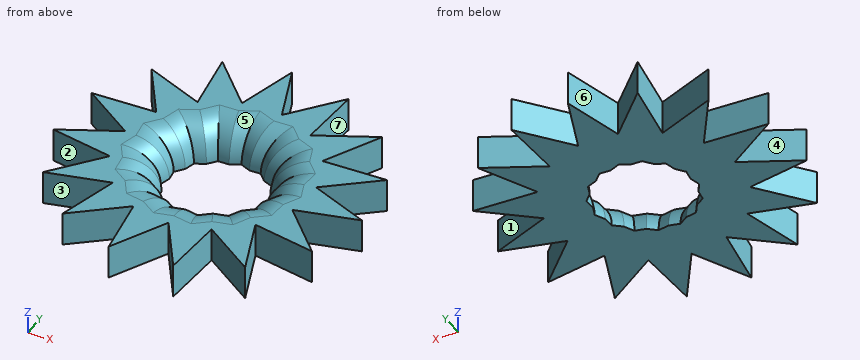
from build123d import *

# Parameters (mm, degrees)
F1_DEPTH = 5.08
F2_R     = 5.07999


# Not quite as in the source:
# - a fillet or chamfer is up to 0.001 mm smaller than in the source, because OpenCascade refuses the exact size


with BuildPart() as f1:
    # F0 (on Top) → F1 (new body)
    with BuildSketch(Plane.XY):
        Polygon((-21.999723834, 5.8521262697), (-14.0514369357, 0.7108895722), (-10.1598827967, 2.7026210629), (-12.5474815477, 6.3646642291), align=None)
        Polygon((-22.4780219717, -3.6019104497), (-13.1257712241, -5.0658043501), (-10.3807697977, -1.6634294271), (-14.0514369357, 0.7108895722), align=None)
        Polygon((-19.0696659041, -12.4331441299), (-9.930540424, -9.9665746788), (-8.8067273944, -5.7418578572), (-13.1257712241, -5.0658043501), align=None)
        Polygon((-9.930540424, -9.9665746788), (-12.3639913592, -19.1145742385), (-5.0182289685, -13.144033702), (-5.7099218179, -8.8274669008), align=None)
        Polygon((-1.6258188862, -10.3867267222), (-5.0182289685, -13.144033702), (-3.5204703849, -22.4909208108), (0.7617798649, -14.0487698884), align=None)
        Polygon((2.7394029011, -10.1500271328), (0.7617798649, -14.0487698884), (5.9317719013, -21.9783828513), (6.4100700391, -12.524346132), align=None)
        Polygon((6.6309570401, -8.1582956421), (6.4100700391, -12.524346132), (14.3583569374, -17.6655828295), (10.9500008698, -8.8343491493), align=None)
        Polygon((9.3759584665, -4.7559207191), (10.9500008698, -8.8343491493), (20.3022516175, -10.2982430497), (13.5965770725, -3.6168129411), align=None)
        Polygon((10.4997714961, -0.5312038976), (13.5965770725, -3.6168129411), (22.7357025527, -1.15024349), (13.8921815784, 2.2261030823), align=None)
        Polygon((9.8080786466, 3.7853629037), (13.8921815784, 2.2261030823), (21.2379439691, 8.1966436188), (11.7857016829, 7.6841056593), align=None)
        Polygon((7.6413668966, 11.8134565599), (7.4204798956, 7.44740607), (11.7857016829, 7.6841056593), (16.0679519327, 16.1262565817), align=None)
        Polygon((8.1196650343, 21.2674932792), (2.1757703543, 13.9001534994), (3.7498127576, 9.8217250692), (7.6413668966, 11.8134565599), align=None)
        Polygon((-1.2325857133, 22.7313871796), (-3.6660366485, 13.5833876199), (-0.5692310721, 10.4977785763), (2.1757703543, 13.9001534994), align=None)
        Polygon((-8.8739526099, 10.9179306197), (-4.7898496782, 9.3586707984), (-3.6660366485, 13.5833876199), (-10.3717111935, 20.2648177285), align=None)
        Polygon((-17.7174735842, 14.294277192), (-12.5474815477, 6.3646642291), (-8.1822597605, 6.6013638185), (-8.8739526099, 10.9179306197), align=None)
        Polygon((-12.5474815477, 6.3646642291), (-10.1598827967, 2.7026210629), (-7.7547700697, 3.9335788206), (-8.1822597605, 6.6013638185), align=None)
        Polygon((-14.0514369357, 0.7108895722), (-10.3807697977, -1.6634294271), (-8.684265617, 0.4393539178), (-10.1598827967, 2.7026210629), align=None)
        Polygon((-13.1257712241, -5.0658043501), (-8.8067273944, -5.7418578572), (-8.112172745, -3.1308392687), (-10.3807697977, -1.6634294271), align=None)
        Polygon((-8.8067273944, -5.7418578572), (-9.930540424, -9.9665746788), (-5.7099218179, -8.8274669008), (-6.1374115087, -6.1596819029), align=None)
        Polygon((-5.7099218179, -8.8274669008), (-5.0182289685, -13.144033702), (-1.6258188862, -10.3867267222), (-3.1014360658, -8.1234595771), align=None)
        Polygon((0.4708058484, -8.6826172912), (-1.6258188862, -10.3867267222), (0.7617798649, -14.0487698884), (2.7394029011, -10.1500271328), align=None)
        Polygon((3.9616411544, -7.7404715965), (2.7394029011, -10.1500271328), (6.4100700391, -12.524346132), (6.6309570401, -8.1582956421), align=None)
        Polygon((6.7674727144, -5.4599280427), (6.6309570401, -8.1582956421), (10.9500008698, -8.8343491493), (9.3759584665, -4.7559207191), align=None)
        Polygon((8.4031467615, -2.2353133286), (9.3759584665, -4.7559207191), (13.5965770725, -3.6168129411), (10.4997714961, -0.5312038976), align=None)
        Polygon((8.5858403933, 1.3758073673), (10.4997714961, -0.5312038976), (13.8921815784, 2.2261030823), (9.8080786466, 3.7853629037), align=None)
        Polygon((7.4204798956, 7.44740607), (7.2839642213, 4.7490384706), (9.8080786466, 3.7853629037), (11.7857016829, 7.6841056593), align=None)
        Polygon((3.7498127576, 9.8217250692), (4.7226244626, 7.3011176786), (7.4204798956, 7.44740607), (7.6413668966, 11.8134565599), align=None)
        Polygon((2.1757703543, 13.9001534994), (-0.5692310721, 10.4977785763), (1.3447000307, 8.5907673114), (3.7498127576, 9.8217250692), align=None)
        Polygon((-3.6660366485, 13.5833876199), (-4.7898496782, 9.3586707984), (-2.2657352528, 8.3949952315), (-0.5692310721, 10.4977785763), align=None)
        Polygon((-8.1822597605, 6.6013638185), (-5.4844043275, 6.7476522098), (-4.7898496782, 9.3586707984), (-8.8739526099, 10.9179306197), align=None)
        Polygon((-10.1598827967, 2.7026210629), (-8.684265617, 0.4393539178), (-7.4416532636, 1.979547329), (-7.7547700697, 3.9335788206), align=None)
        Polygon((-10.3807697977, -1.6634294271), (-8.112172745, -3.1308392687), (-7.6034429717, -1.2183865968), (-8.684265617, 0.4393539178), align=None)
        Polygon((-8.112172745, -3.1308392687), (-8.8067273944, -5.7418578572), (-6.1374115087, -6.1596819029), (-6.4505283149, -4.2056504113), align=None)
        Polygon((-6.1374115087, -6.1596819029), (-5.7099218179, -8.8274669008), (-3.1014360658, -8.1234595771), (-4.1822587112, -6.4657190625), align=None)
        Polygon((-3.1014360658, -8.1234595771), (-1.6258188862, -10.3867267222), (0.4708058484, -8.6826172912), (-1.1908385817, -7.6078061486), align=None)
        Polygon((2.0064883569, -7.4344344369), (0.4708058484, -8.6826172912), (2.7394029011, -10.1500271328), (3.9616411544, -7.7404715965), align=None)
        Polygon((4.8568752303, -5.9755814713), (3.9616411544, -7.7404715965), (6.6309570401, -8.1582956421), (6.7674727144, -5.4599280427), align=None)
        Polygon((6.867464253, -3.4834961829), (6.7674727144, -5.4599280427), (9.3759584665, -4.7559207191), (8.4031467615, -2.2353133286), align=None)
        Polygon((7.6906063175, -0.3890827578), (8.4031467615, -2.2353133286), (10.4997714961, -0.5312038976), (8.5858403933, 1.3758073673), align=None)
        Polygon((7.2839642213, 4.7490384706), (7.1839726826, 2.7726066107), (8.5858403933, 1.3758073673), (9.8080786466, 3.7853629037), align=None)
        Polygon((4.7226244626, 7.3011176786), (5.4351649066, 5.4548871079), (7.2839642213, 4.7490384706), (7.4204798956, 7.44740607), align=None)
        Polygon((-0.5692310721, 10.4977785763), (-2.2657352528, 8.3949952315), (-0.4169359382, 7.6891465941), (1.3447000307, 8.5907673114), align=None)
        Polygon((-4.7898496782, 9.3586707984), (-5.4844043275, 6.7476522098), (-3.5083476063, 6.8548018203), (-2.2657352528, 8.3949952315), align=None)
        Polygon((-7.4416532636, 1.979547329), (-6.4138998748, 3.2534273071), (-5.9931341009, 4.8351995379), (-7.7547700697, 3.9335788206), align=None)
        Polygon((-8.684265617, 0.4393539178), (-7.6034429717, -1.2183865968), (-7.1826771978, 0.363385634), (-7.4416532636, 1.979547329), align=None)
        Polygon((-7.6034429717, -1.2183865968), (-8.112172745, -3.1308392687), (-6.4505283149, -4.2056504113), (-6.7095043807, -2.5894887164), align=None)
        Polygon((-6.4505283149, -4.2056504113), (-6.1374115087, -6.1596819029), (-4.1822587112, -6.4657190625), (-5.0761973022, -5.0946169429), align=None)
        Polygon((-4.1822587112, -6.4657190625), (-3.1014360658, -8.1234595771), (-1.1908385817, -7.6078061486), (-2.5651695944, -6.7188396169), align=None)
        Polygon((-1.1908385817, -7.6078061486), (0.4708058484, -8.6826172912), (2.0064883569, -7.4344344369), (0.3893992401, -7.1813138824), align=None)
        Polygon((3.2766374084, -6.4020737375), (2.0064883569, -7.4344344369), (3.9616411544, -7.7404715965), (4.8568752303, -5.9755814713), align=None)
        Polygon((5.5973152015, -4.5158568823), (4.8568752303, -5.9755814713), (6.7674727144, -5.4599280427), (6.867464253, -3.4834961829), align=None)
        Polygon((6.9501663462, -1.8488073469), (6.867464253, -3.4834961829), (8.4031467615, -2.2353133286), (7.6906063175, -0.3890827578), align=None)
        Polygon((7.1839726826, 2.7726066107), (7.1012705894, 1.1379177747), (7.6906063175, -0.3890827578), (8.5858403933, 1.3758073673), align=None)
        Polygon((1.3447000307, 8.5907673114), (2.7465677414, 7.1939680681), (4.7226244626, 7.3011176786), (3.7498127576, 9.8217250692), align=None)
        Polygon((4.7226244626, 7.3011176786), (2.7465677414, 7.1939680681), (3.9060397893, 6.0386881034), (5.4351649066, 5.4548871079), align=None)
        Polygon((-0.4169359382, 7.6891465941), (1.1121891791, 7.1053455986), (2.7465677414, 7.1939680681), (1.3447000307, 8.5907673114), align=None)
        Polygon((-2.2657352528, 8.3949952315), (-3.5083476063, 6.8548018203), (-1.873969044, 6.9434242898), (-0.4169359382, 7.6891465941), align=None)
        Polygon((-5.4844043275, 6.7476522098), (-5.9931341009, 4.8351995379), (-4.536100995, 5.5809218422), (-3.5083476063, 6.8548018203), align=None)
        Polygon((-7.7547700697, 3.9335788206), (-5.9931341009, 4.8351995379), (-5.4844043275, 6.7476522098), (-8.1822597605, 6.6013638185), align=None)
        Polygon((5.4351649066, 5.4548871079), (6.0245006347, 3.9278865754), (7.1839726826, 2.7726066107), (7.2839642213, 4.7490384706), align=None)
    extrude(amount=F1_DEPTH)

    # F2 (radius 5.08 in the source; OpenCascade refuses exactly that, so slightly less here)
    f2_edges = [f1.edges().sort_by_distance(p)[0] for p in [
        (-6.203517, 4.044313, 5.08),
        (-6.927777, 2.616487, 5.08),
        (-7.312165, 1.171466, 5.08),
        (-7.39306, -0.4275, 5.08),
        (-7.156474, -1.903938, 5.08),
        (-6.580016, -3.39757, 5.08),
        (-5.763363, -4.650134, 5.08),
        (-4.629228, -5.780168, 5.08),
        (-3.373714, -6.592279, 5.08),
        (-1.878004, -7.163323, 5.08),
        (-0.40072, -7.39456, 5.08),
        (1.197944, -7.307874, 5.08),
        (2.641563, -6.918254, 5.08),
        (4.066756, -6.188828, 5.08),
        (5.227095, -5.245719, 5.08),
        (6.908815, -2.666152, 5.08),
        (7.320386, -1.118945, 5.08),
        (7.395938, 0.374418, 5.08),
        (7.142622, 1.955262, 5.08),
        (6.604237, 3.350247, 5.08),
        (3.326304, 6.616328, 5.08),
        (5.729833, 4.691387, 5.08),
        (4.670602, 5.746788, 5.08),
        (1.929378, 7.149657, 5.08),
        (0.347627, 7.397246, 5.08),
        (-1.145452, 7.316285, 5.08),
        (-2.691158, 6.899113, 5.08),
        (-4.022224, 6.217862, 5.08),
        (-5.264618, 5.208061, 5.08),
        (6.23239, -3.999677, 5.08),
    ]]
    fillet(f2_edges, radius=F2_R)


solid = f1.part
Part model, mm, in its own coordinate system. Face numbers are marked on the shaded views. A direction names the side the tool comes from. Coordinates: 2 decimals unless noted, no trailing zeros. Loops run counter-clockwise (first coordinate to the right, second up) from the corner with the lowest first, then second, coordinate; pieces in that order, holes last. Notation, with made-up numbers: (80, 27.5) - (117, 27.5) arc R32 cw to (117, 54.5) - close; hole circle Ø1 at (52.5, -24.5). An arc over 180 degrees is marked (long way). Write each question's results on one line, items separated by ' | '. Start each with the question number.
Q1. Which spindle directions (+Z, -Z, +X, -X, +Y, -Y) get a long thin tool onto all of the face, cutting with end or side? Do the marked faces 4, 5, 6 and 7. Say none if no direction does.
Q2. Slice it at B-B on y = -17. Give the cut face in (x, z), and give its area (3 significant figures).
Q3. Two-plate mould, pull along X, no slides. Class the marked faces 1, 2 and 3: +X half, -X half, draft (parallel to the pull), parting line (faces both ways), or undercut.
Q4. Probe line 1 along X through (y, z) = (-16, 3.5); line 2 along Y through (x, z) = (-19.5, 1.7); line 3 along Y through (x, z) = (3, 1.65). List the from-to ranges inside material, lowest first.
Q5. Slice it at A-A on x = -17. Give the cut face in (y, z).
Q6. Drop flat-ended pins along their axis: pin 1 Ø3 at (x, z) = (7.5, 1) entering from +Y; pin 2 Ø1 at (x, z) = (0.5, 2) entering from -Y; pin 3 Ø1.5 at (x, z) = (3.5, 3.5) entering from -Y. Give the stop position or say it passes through.
Answer:
1) face 4: +Z, -Z, -X | face 5: +Z | face 6: +Z, -Z, +Y | face 7: +Z, -Z
2) outline: (-11.8, 0) - (-9.76, 0) - (-9.76, 5.08) - (-11.8, 5.08) - close; (-4.4, 0) - (-0.74, 0) - (-0.74, 5.08) - (-4.4, 5.08) - close; (2.69, 0) - (6.18, 0) - (6.18, 5.08) - (2.69, 5.08) - close; (13.33, 0) - (14.1, 0) - (14.1, 5.08) - (13.33, 5.08) - close | area: 50.7 mm2
3) face 1: +X half | face 2: -X half | face 3: undercut
4) line 1: x = -11.54 to -8.53, -4.56 to -0.23, 2.03 to 6.23, 11.78 to 13.72 | line 2: y = -4.07 to -2.08, 4.24 to 5.99 | line 3: y = -17.48 to -6.98, 7.33 to 14.92
5) outline: (-11.87, 0) - (-9.87, 0) - (-9.87, 5.08) - (-11.87, 5.08) - close; (-4.46, 0) - (-0.8, 0) - (-0.8, 5.08) - (-4.46, 5.08) - close; (2.62, 0) - (6.12, 0) - (6.12, 5.08) - (2.62, 5.08) - close; (13.19, 0) - (14.02, 0) - (14.02, 5.08) - (13.19, 5.08) - close
6) pin 1: stops at y = 21.27 | pin 2: stops at y = -15.55 | pin 3: stops at y = -19.4
